Read the model definition and answer for the solid it produces. Units are mm, in the model's axes. A direction names the side the tool comes from. Round coordinates to 2 decimals unless told otherwise and drop trailing zeros. Loops run counter-clockwise (first coordinate to the right, second up) from the corner with the lowest first, then second, coordinate; pieces in that order, holes last. Notation, with made-up numbers: M -6.5,48.25 L 20.5,48.25 A20 ccw 20.5,74.25 Z; hole C 69,-16.75 d9. An arc over 180 degrees is marked long. Write each question's results on one line, items separated by ' | '.
Autodesk Inventor part; units mm, degrees
ref_plane "YZ Plane" through (0, 0, 0) normal (1, 0, 0) x (0, 1, 0)
ref_plane "XZ Plane" through (0, 0, 0) normal (0, 1, 0) x (-1, 0, 0)
ref_plane "XY Plane" through (0, 0, 0) normal (0, 0, 1) x (1, 0, 0)
sketch "Sketch1" plane through (0, 0, 0) normal (0, 0, 1) x (1, 0, 0)
  line L0 (0, 0) -> (50.8, 0)
  line L1 (50.8, 0) -> (50.8, -50.8)
  line L2 (50.8, -50.8) -> (0, -50.8)
  line L3 (0, -50.8) -> (0, 0)
  circle A0 centre (25.4, -25.4) radius 9.5885
  line L4 (0, -50.8) -> (-12.7, -50.8)
  line L5 (-12.7, -50.8) -> (-12.7, 50.8)
  line L6 (-12.7, 50.8) -> (-6.35, 50.8)
  line L7 (0, 0) -> (0, -50.8)
  line L8 (50.8, -50.8) -> (63.5, -50.8)
  line L9 (63.5, -50.8) -> (63.5, 50.8)
  line L10 (63.5, 50.8) -> (57.15, 50.8)
  line L11 (50.8, 0) -> (50.8, -50.8)
  line L12 (-6.35, 50.8) -> (-6.35, 0)
  line L13 (-6.35, 0) -> (0, 0)
  line L14 (57.15, 50.8) -> (57.15, 0)
  line L15 (57.15, 0) -> (50.8, 0)
  dimension "d0" = 19.177
  dimension "d1" = 50.8
  dimension "d2" = 50.8
  dimension "d37" = 25.4
  dimension "d44" = 101.6
  dimension "d45" = 101.6
extrude "Extrusion1" add sketch "Sketch1" against normal blind 12.7
sketch "Sketch9" plane through (63.5, -50.8, 0) normal (1, 0, 0) x (0, 0, -1)
  line L0 (0, 101.6) -> (0, 0)
  line L1 (0, 101.6) -> (12.7, 101.6)
  circle A0 centre (6.35, 76.2) radius 2.4447
  point P0 (0, 50.8)
  dimension "d48" = 4.8895
  dimension "d49" = 6.35
  dimension "d50" = 25.4
extrude "Extrusion9" cut sketch "Sketch9" against normal through all
fillet "Fillet13" radius 1.5875 4 edges at (-12.7, 50.8, -6.35) (-6.35, 50.8, -6.35) (57.15, 50.8, -6.35) (63.5, 50.8, -6.35)
fillet "Fillet14" radius 6.35 4 edges at (63.5, -50.8, -6.35) (-12.7, -50.8, -6.35) (-6.35, 0, -6.35) (57.15, 0, -6.35)
properties part number "Needle Bearing Mount" material "ABS Plastic"
1. Find section A-A, the plane z = -6.35. Count the separate pieces of the cut face and the enclosed holes in it, then the cut area to 3 significant figures.
Completed:
separate pieces: 3 | enclosed holes: 1 | area: 4,160 mm2
2. Which of the six approach directions +Z, -Z, +X, -X, +Y, -Y give full straight-line access (tool end or side, diameter ignored) to faces 5 (the face through (55.34, 1.91, -6.44)), 6 (the face through (25, -11, 0))?
Completed:
face 5: +Z, -Z, +Y | face 6: +Z, +X, -X, +Y, -Y
3. Given P1, Ø3, axis at x = 52, z = -3.5, coming from the +Y side, flat-ended and moving along its own axis, determine where the tip first touches the part or whether it passes through.
Completed:
P1: stops at y = 0.6
4. Find section C-C, the plane x = 25.4. Give the vertices of the cut face in (y, z), then the cut area to 3 significant figures.
Completed:
outline: M -50.8,-12.7 L -34.99,-12.7 L -34.99,0 L -50.8,0 Z; M -15.81,-12.7 L 0,-12.7 L 0,0 L -15.81,0 Z | area: 402 mm2
5. Find the intervals of material crossed by L1, parallel to X at y = 45, z = -10.5; L2, parallel to Y at x = 43.5, z = -3.25; L3, parallel to Y at x = 25.4, z = -5, in increasing order.
Completed:
L1: x = -12.7 to -6.35, 57.15 to 63.5 | L2: y = -50.8 to 0 | L3: y = -50.8 to -34.99, -15.81 to 0
6. Find section B-B, the plane y = -25.4. Give the vertices of the cut face in (x, z).
Completed:
outline: M -12.7,-12.7 L 15.81,-12.7 L 15.81,0 L -12.7,0 Z; M 34.99,-12.7 L 63.5,-12.7 L 63.5,0 L 34.99,0 Z
7. Determine the mould class of faces 1 (the face through (61.69, -48.89, -6.44)), 2 (the face through (-6.35, 28, -6)), 3 (the face through (17.79, -31.23, -6.26)), 4 (the face through (60, 50.8, -6)) for opening direction Y: released by +Y, released by -Y, zero draft, split by the parting line, or undercut.
Completed:
face 1: released by -Y | face 2: zero draft | face 3: undercut | face 4: released by +Y
8. Find section D-D, the plane y = 25.4. Give the vertices of the cut face in (x, z), then the cut area to 3 significant figures.
Completed:
outline: M -12.7,-12.7 L -6.35,-12.7 L -6.35,-8.79 L -12.7,-8.79 Z; M -12.7,-3.91 L -6.35,-3.91 L -6.35,0 L -12.7,0 Z; M 57.15,-12.7 L 63.5,-12.7 L 63.5,-8.79 L 57.15,-8.79 Z; M 57.15,-3.91 L 63.5,-3.91 L 63.5,0 L 57.15,0 Z | area: 99.2 mm2
